from build123d import *

# Parameters (mm, degrees)
SKETCH1_W           = 70
SKETCH1_H           = 42.5
BOSS_EXTRUDE1_DEPTH = 2
SKETCH2_W           = 66
SKETCH2_H           = 38.5
SKETCH2_W_2         = 62
SKETCH2_H_2         = 34.5
BOSS_EXTRUDE2_DEPTH = 11
FILLET1_R           = 1
SKETCH3_R           = 5
CUT_EXTRUDE1_DEPTH  = 0.5


with BuildPart() as part:
    # Sketch1 → Boss-Extrude1 (new body)
    with BuildSketch(Plane(origin=(0, 0, 0), x_dir=(1, 0, 0), z_dir=(0, 1, 0))):
        Rectangle(SKETCH1_W, SKETCH1_H)
    extrude(amount=-BOSS_EXTRUDE1_DEPTH)

    # Sketch2 → Boss-Extrude2 (add)
    with BuildSketch(Plane(origin=(0, 0, 0), x_dir=(-1, 0, 0), z_dir=(0, 1, 0))):
        Rectangle(SKETCH2_W, SKETCH2_H)
        Rectangle(SKETCH2_W_2, SKETCH2_H_2, mode=Mode.SUBTRACT)
    extrude(amount=BOSS_EXTRUDE2_DEPTH)

    # Fillet1
    fillet1_edges = [part.edges().sort_by_distance(p)[0] for p in [
        (35, -2, 0),
        (0, -2, -21.25),
        (0, 0, -17.25),
        (-31, 5.5, -17.25),
        (31, 0, 0),
        (31, 5.5, -17.25),
        (0, 11, 17.25),
        (31, 5.5, 17.25),
        (-33, 5.5, 19.25),
        (33, 5.5, 19.25),
        (0, 11, -19.25),
        (33, 5.5, -19.25),
        (-33, 11, 0),
        (-33, 5.5, -19.25),
        (-31, 11, 0),
        (-31, 5.5, 17.25),
        (0, 11, 19.25),
        (33, 11, 0),
        (0, 11, -17.25),
        (31, 11, 0),
        (-31, 0, 0),
        (0, 0, 17.25),
        (-35, -2, 0),
        (-35, -1, -21.25),
        (35, -1, -21.25),
        (35, -1, 21.25),
        (-35, -1, 21.25),
        (0, -2, 21.25),
    ]]
    fillet(fillet1_edges, radius=FILLET1_R - 0.0001)  # a hair under: the kernel refuses the full size

    # Sketch3 → Cut-Extrude1 (cut)
    with BuildSketch(Plane.XZ.offset(2)):
        with BuildLine():
            ThreePointArc((12.000000021, 8.999999972), (8.499999983, 9.499999987), (8.000000047, 5.999999937))
            ThreePointArc((8.000000047, 5.999999937), (10, -3.8e-08), (8.000000001, -5.999999998))
            ThreePointArc((8.000000001, -5.999999998), (8.499999982, -9.499999987), (11.999999975, -9.000000033))
            ThreePointArc((11.999999975, -9.000000033), (15, -3.8e-08), (12.000000021, 8.999999972))
        make_face()
        with Locations(Location((0, 0, 0), (0, 0, 270))):
            Circle(SKETCH3_R)
        with BuildLine():
            ThreePointArc((-8.000000081, -5.999999892), (-10, -1.9e-08), (-8.000000104, 5.999999861))
            ThreePointArc((-8.000000104, 5.999999861), (-8.499999944, 9.499999958), (-12.000000021, 8.999999972))
            ThreePointArc((-12.000000021, 8.999999972), (-15, 3.8e-08), (-12.000000067, -8.999999911))
            ThreePointArc((-12.000000067, -8.999999911), (-8.49999999, -9.499999993), (-8.000000081, -5.999999892))
        make_face()
        with BuildLine():
            ThreePointArc((16.62958836, 11.111111149), (20, -3.3e-08), (16.629588323, -11.111111204))
            ThreePointArc((16.629588323, -11.111111204), (17.319398074, -14.578698568), (20.786985459, -13.888888924))
            ThreePointArc((20.786985459, -13.888888924), (25, -2.4e-08), (20.786985486, 13.888888883))
            ThreePointArc((20.786985486, 13.888888883), (17.319398067, 14.578698563), (16.62958836, 11.111111149))
        make_face()
        with BuildLine():
            ThreePointArc((-16.629588323, -11.111111204), (-20, 2.3e-08), (-16.629588298, 11.111111242))
            ThreePointArc((-16.629588298, 11.111111242), (-17.319398098, 14.578698584), (-20.786985465, 13.888888914))
            ThreePointArc((-20.786985465, 13.888888914), (-25, -1.1e-08), (-20.786985453, -13.888888933))
            ThreePointArc((-20.786985453, -13.888888933), (-17.31939807, -14.578698565), (-16.629588323, -11.111111204))
        make_face()
    extrude(amount=-CUT_EXTRUDE1_DEPTH, mode=Mode.SUBTRACT)


solid = part.part
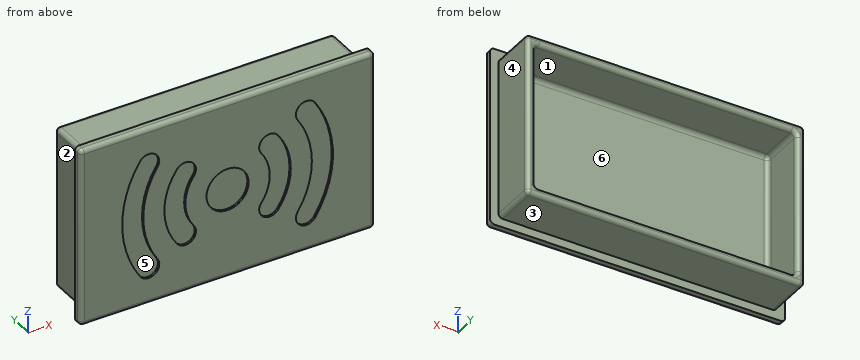
CAD build for the part. Positions are in the model's coordinates, mm. Face numbers are marked on the shaded views. A direction names the side the tool comes from. Round coordinates to 2 decimals unless told otherwise and drop trailing zeros. Loops run counter-clockwise (first coordinate to the right, second up) from the corner with the lowest first, then second, coordinate; pieces in that order, holes last. Notation, with made-up numbers: M 60.5,-14.5 L 98.5,-14.5 A5 cw 98.5,-5.5 Z; hole C 57.5,14.25 d7. An arc over 180 degrees is marked long. One line per question, with ' | ' between items. Start each with the question number.
Item 1: Cut at A-A, the plane y = 4. Write the cut outline in (x, z), plus the area to 3 significant figures.
Item 2: Two-plate mould, pull along X, no slides. Class the marked faces 1, 2 and 3: pulls with the +X half, pulls with the -X half, needs draft (parallel to the pull), parting line crosses it, or undercut.
Item 3: Wall check: line 1 (X direction, y = 3.5, z = -1); line 2 (Z direction, x = 12, y = 1); line 3 (Y direction, x = 16.5, z = 11). Give the ranges that are in metal, low to high.
Item 4: Which spindle directions (+Z, -Z, +X, -X, +Y, -Y) get a long thin tool onto all of the face, cutting with end or side? Do the marked faces 4, 5 and 6. Say none if no direction does.
Item 5: Pin check, flat tips, straight feed: pin 1 Ø5 at (x, y) = (-10.5, 3.5) entering from -Z; pin 2 Ø6 at (y, z) = (9.5, 0) entering from -X; pin 3 Ø10 at (x, z) = (18.5, -4.5) entering from +Y. Stop position of each tip, or through.
Responses:
1) outline: M -33,-18.25 A1 ccw -32,-19.25 L 32,-19.25 A1 ccw 33,-18.25 L 33,18.25 A1 ccw 32,19.25 L -32,19.25 A1 ccw -33,18.25 Z; hole M -31,-16.25 A1 ccw -30,-17.25 L 30,-17.25 A1 ccw 31,-16.25 L 31,16.25 A1 ccw 30,17.25 L -30,17.25 A1 ccw -31,16.25 Z | area: 402 mm²
2) face 1: undercut | face 2: pulls with the -X half | face 3: needs draft
3) line 1: x = -33 to -31, 31 to 33 | line 2: z = -19.25 to -17.25, 17.25 to 19.25 | line 3: y = -2 to 0
4) face 4: +Z, -Z, +X, +Y | face 5: -Y | face 6: +Y
5) pin 1: stops at z = -19.25 | pin 2: stops at x = -33 | pin 3: stops at y = 0
